Design review of the part built by this model. Coordinates are the model's own, in mm. Face numbers are marked on the shaded views. A direction names the side the tool comes from. Round coordinates to 2 decimals unless told otherwise and drop trailing zeros. Order: outer loops, then holes, each group sorted by start corner. A loop starts at its lowest first (then second) coordinate and runs counter-clockwise, first axis right, second up. Notation, with made-up numbers: M 64.25,-29 L 76.25,-29 A20 ccw 76.25,-23 Z; hole C 22,-1 d8. An arc over 180 degrees is marked long. Use a Markdown table: item, result. Add a question column.
(1) Machinability: for the marked faces 1, 2 and 3, which of the approach directions +Z, -Z, +X, -X, +Y, -Y give a long, thin tool a straight path to every point of the face, cutting with its end or side? Answer none if there is none.
(2) Take a section at C-C (x = 2.75). Write out the cut boundary in (y, z).
(3) For pin 1 (4 mm diameter, centred on y = 0, z = -8, fed in from +X); pin 2 (1 mm diameter, centred on y = -4, z = -8.5, fed in from -X); pin 3 (2 mm diameter, centred on x = 7.5, y = -0.5, fed in from +Z), all flat-tipped, find the tip position at first contact; note any pin that passes through.
(4) Take a section at A-A (y = 0). Write out the cut boundary in (x, z), then the cut area to 3 significant figures.
(5) To check wall thickness, follow probe 1 along X at (y, z) = (-2, 4.75); probe 2 along Y at (x, z) = (6.25, 0); probe 3 along Z at (x, y) = (2.75, 0.5). State the ranges of each line that lie inside material, in increasing order. Write a range as from..to.
(6) The part is to be moulded in two halves that separate along Z. For the marked faces 4, 5 and 6, say which applies: released by +Z, released by -Z, zero draft, split by the parting line, or undercut.
(7) Take a section at D-D (y = 2.25). Write out the cut boundary in (x, z), then the cut area to 3 significant figures.
(8) Take a section at B-B (z = 0). Write out the cut boundary in (x, y).
```python
from build123d import *

# Parameters (mm, degrees)
SKETCH_1_R      = 5
SKETCH_1_R_2    = 4
EXTRUDE_1_DEPTH = 1.5
SKETCH_2_R      = 4
SKETCH_2_R_2    = 1.75
EXTRUDE_2_DEPTH = 3.5
SKETCH_3_R      = 5
SKETCH_3_R_2    = 4
EXTRUDE_3_DEPTH = 10


with BuildPart() as part:
    # 草图1 → 凸台-拉伸1 (new body)
    with BuildSketch(Plane(origin=(0, 0, 0), x_dir=(0, 0, -1), z_dir=(1, 0, 0))):
        Circle(SKETCH_1_R)
        Circle(SKETCH_1_R_2, mode=Mode.SUBTRACT)
    extrude(amount=EXTRUDE_1_DEPTH)

    # 草图2 → 凸台-拉伸2 (add)
    with BuildSketch(Plane(origin=(1.5, 0, 0), x_dir=(0, 0, -1), z_dir=(1, 0, 0))):
        with BuildLine():
            Line((-9.746281342, 5.1), (9.746281342, 5.1))
            ThreePointArc((9.746281342, 5.1), (11, 0), (9.746281342, -5.1))
            Line((9.746281342, -5.1), (-9.746281342, -5.1))
            ThreePointArc((-9.746281342, -5.1), (-11, 0), (-9.746281342, 5.1))
        make_face()
        Circle(SKETCH_2_R, mode=Mode.SUBTRACT)
        with Locations((-8, 0)):
            Circle(SKETCH_2_R_2, mode=Mode.SUBTRACT)
        with Locations((8, 0)):
            Circle(SKETCH_2_R_2, mode=Mode.SUBTRACT)
    extrude(amount=EXTRUDE_2_DEPTH)

    # 草图3 → 凸台-拉伸3 (add)
    with BuildSketch(Plane(origin=(5, 0, 0), x_dir=(0, 0, -1), z_dir=(1, 0, 0))):
        Circle(SKETCH_3_R)
        Circle(SKETCH_3_R_2, mode=Mode.SUBTRACT)
    extrude(amount=EXTRUDE_3_DEPTH)


solid = part.part
```
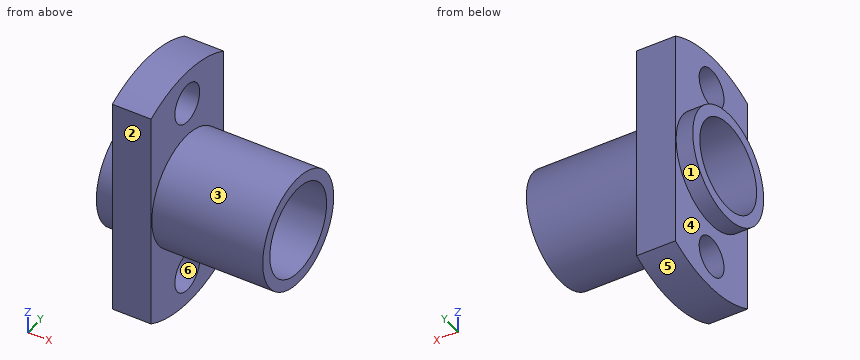
Verdict:
| question | item | result |
|---|---|---|
| 1 | face 1 | -X |
| 1 | face 2 | +Z, -Z, +X, -X, -Y |
| 1 | face 3 | +X |
| 2 | outline | M -5.1,-9.75 A11 ccw 5.1,-9.75 L 5.1,9.75 A11 ccw -5.1,9.75 Z; hole C 0,0 d8; hole C 0,-8 d3.5; hole C 0,8 d3.5 |
| 3 | pin 1 | stops at x = 5 |
| 3 | pin 2 | stops at x = 1.5 |
| 3 | pin 3 | stops at z = 5 |
| 4 | outline | M 0,-5 L 1.5,-5 L 1.5,-6.25 L 5,-6.25 L 5,-5 L 15,-5 L 15,-4 L 0,-4 Z; M 0,4 L 15,4 L 15,5 L 5,5 L 5,6.25 L 1.5,6.25 L 1.5,5 L 0,5 Z; M 1.5,-11 L 5,-11 L 5,-9.75 L 1.5,-9.75 Z; M 1.5,9.75 L 5,9.75 L 5,11 L 1.5,11 Z |
| 4 | area | 47.5 mm^2 |
| 5 | probe 1 | x = 1.5..5 |
| 5 | probe 2 | y = -5..-4, 4..5 |
| 5 | probe 3 | z = -10.99..-9.68, -6.32..-3.97, 3.97..6.32, 9.68..10.99 |
| 6 | face 4 | zero draft |
| 6 | face 5 | released by -Z |
| 6 | face 6 | undercut |
| 7 | outline | M 0,-4.47 L 1.5,-4.47 L 1.5,-10.77 L 5,-10.77 L 5,-4.47 L 15,-4.47 L 15,-3.31 L 0,-3.31 Z; M 0,3.31 L 15,3.31 L 15,4.47 L 5,4.47 L 5,10.77 L 1.5,10.77 L 1.5,4.47 L 0,4.47 Z |
| 7 | area | 78.9 mm^2 |
| 8 | outline | M 0,-5 L 1.5,-5 L 1.5,-5.1 L 5,-5.1 L 5,-5 L 15,-5 L 15,-4 L 0,-4 Z; M 0,4 L 15,4 L 15,5 L 5,5 L 5,5.1 L 1.5,5.1 L 1.5,5 L 0,5 Z |
